Check sheet for the modelled part. Datum: model origin and axes. Units: mm. Round coordinates to 2 decimals unless told otherwise and drop trailing zeros. Write each loop counter-clockwise with the first axis right and the second up, starting at its lowest first coordinate (ties: lowest second). Pieces come first, ordered by that corner, then holes.
Item 1: Release check for a two-part mould opening along Z. For faces 1 (the flat face through (-3, -1, 0)), 2 (the cylindrical face through (10.24, -23.84, 17.01)) record: +Z half, -Z half, draft (parallel to the pull), parting line (faces both ways), or undercut.
Item 2: Go/stop test with flat-tipped pins: pin 1 Ø6 at (y, z) = (8, 27) entering from +X; pin 2 Ø5 at (y, z) = (12, 13.5) entering from -X; pin 3 Ø3 at (x, y) = (-8.5, 27.5) entering from -Z; pin 4 Ø1 at (x, z) = (25, 6.5) entering from -Y. Record where each tip stops, or that it passes through.
Item 3: Material ranges on line 1 (X direction, y = -22, z = 17); line 2 (Z direction, x = -1, y = -18.5); line 3 (Y direction, x = 5, z = 26.5), recorded low to high.
Item 4: Cross-section at A-A on z = 11.5. Enter the section's corners in (x, y).
Item 5: Cross-section at B-B on z = 16.5. Enter the section's corners in (x, y), plus the area to 3 significant figures.
from build123d import *

# Parameters (mm, degrees)
F1_DEPTH    = 30
F2_T1_DEPTH = 201.5265861528
F2_T3_DEPTH = 201.5265861528
F2_T5_DEPTH = 201.5265861528
F2_T7_DEPTH = 201.5265861528
F2_T9_DEPTH = 201.5265861528


# Not quite as in the source:
# - a fillet or chamfer that OpenCascade refuses, or shapes differently, is made with other operations: its cross-section is extruded or revolved along the edge and cut away or added


with BuildPart() as f1:
    # F0 (on Top) → F1 (new body)
    with BuildSketch(Plane.XY):
        Polygon((-15.9371768066, 35.8527074811), (-39.0228095523, -4.0780599472), (-8.1802458333, -38.3730871366), (33.967139591, -19.6378121565), (29.1730926011, 26.2362517592), align=None)
    extrude(amount=F1_DEPTH)

    # F2: fillet of radius 31.1 on 5 edges, made by hand

    # F2_s2 → F2_t1 (cut)
    with BuildSketch(Plane(origin=(50.4334024594, 87.2336698068, 0), x_dir=(0, 0, 1), z_dir=(-0.5005136386, -0.8657286512, 0))):
        with BuildLine():
            ThreePointArc((0, 31.7420396575), (21.2765502256, 22.2601101881), (30, 0.6614991217))
            Line((30, 0.6614991217), (30, 31.7420396575))
            Line((30, 31.7420396575), (0, 31.7420396575))
        make_face()
    extrude(amount=F2_T1_DEPTH, mode=Mode.SUBTRACT)

    # F2_s4 → F2_t3 (cut)
    with BuildSketch(Plane(origin=(-67.379371666, 74.9217025, 0), x_dir=(0, 0, 1), z_dir=(0.6686896548, -0.7435416233, 0))):
        with BuildLine():
            ThreePointArc((0, 31.7420396575), (21.2765502256, 22.2601101881), (30, 0.6614991217))
            Line((30, 0.6614991217), (30, 31.7420396575))
            Line((30, 31.7420396575), (0, 31.7420396575))
        make_face()
    extrude(amount=F2_T3_DEPTH, mode=Mode.SUBTRACT)

    # F2_s6 → F2_t5 (cut)
    with BuildSketch(Plane(origin=(-92.0761442896, -40.9295111669, 0), x_dir=(0, 0, 1), z_dir=(0.9137865732, 0.406194656, 0))):
        with BuildLine():
            ThreePointArc((0, 31.7420396575), (21.2765502256, 22.2601101881), (30, 0.6614991217))
            Line((30, 0.6614991217), (30, 31.7420396575))
            Line((30, 31.7420396575), (0, 31.7420396575))
        make_face()
    extrude(amount=F2_T5_DEPTH, mode=Mode.SUBTRACT)

    # F2_s8 → F2_t7 (cut)
    with BuildSketch(Plane(origin=(10.473184942, -100.217531544, 0), x_dir=(0, 0, 1), z_dir=(-0.1039384941, 0.9945837267, 0))):
        with BuildLine():
            ThreePointArc((0, 31.7420396575), (21.2765502256, 22.2601101881), (30, 0.6614991217))
            Line((30, 0.6614991217), (30, 31.7420396575))
            Line((30, 31.7420396575), (0, 31.7420396575))
        make_face()
    extrude(amount=F2_T7_DEPTH, mode=Mode.SUBTRACT)

    # F2_s10 → F2_t9 (cut)
    with BuildSketch(Plane(origin=(98.5489285542, -21.0083295959, 0), x_dir=(0, 0, 1), z_dir=(-0.9780240953, 0.2084918918, 0))):
        with BuildLine():
            ThreePointArc((0, 31.7420396575), (21.2765502256, 22.2601101881), (30, 0.6614991217))
            Line((30, 0.6614991217), (30, 31.7420396575))
            Line((30, 31.7420396575), (0, 31.7420396575))
        make_face()
    extrude(amount=F2_T9_DEPTH, mode=Mode.SUBTRACT)


solid = f1.part
Response values:
1. face 1: -Z half
1. face 2: +Z half
2. pin 1: stops at x = 18.3
2. pin 2: stops at x = -27.57
2. pin 3: stops at z = 0
2. pin 4: stops at y = -22.87
3. line 1: x = -15.12 to 14.4
3. line 2: z = 0 to 25.67
3. line 3: y = -14.19 to 14.27
4. outline: (-35.77, -3.74) - (-7.5, -35.17) - (31.13, -18) - (26.74, 24.05) - (-14.61, 32.86) - close
5. outline: (-32.34, -3.38) - (-6.78, -31.8) - (28.15, -16.27) - (24.17, 21.74) - (-13.21, 29.71) - close
5. area: 2,510 mm2
